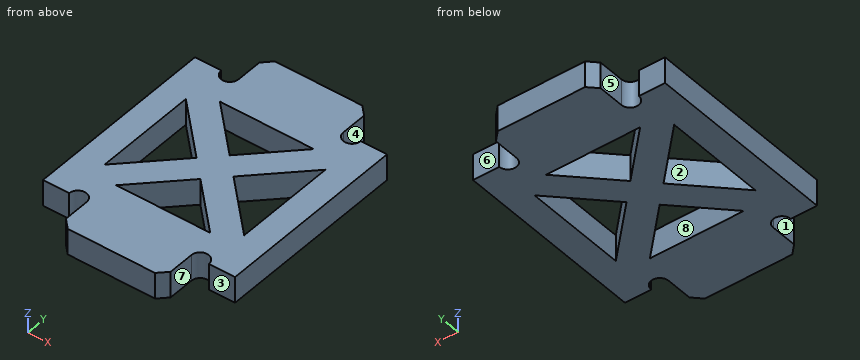
```python
from build123d import *

# Parameters (mm, degrees)
EXTRUDE_1_DEPTH = 1.5
CHAMFER_1_SIZE  = 1


with BuildPart() as part:
    # 草图1 → 凸台-拉伸1 (new, symmetric)
    with BuildSketch(Plane.XY):
        with BuildLine():
            Line((-6, 15), (-6, 11))
            ThreePointArc((-6, 11), (-7, 10), (-8, 11))
            Line((-8, 11), (-11, 11))
            Line((-11, 11), (-11, -11))
            Line((-11, -11), (-8, -11))
            ThreePointArc((-8, -11), (-7, -10), (-6, -11))
            Line((-6, -11), (-6, -15))
            Line((-6, -15), (6, -15))
            Line((6, -15), (6, -11))
            ThreePointArc((6, -11), (7, -10), (8, -11))
            Line((8, -11), (11, -11))
            Line((11, -11), (11, 11))
            Line((11, 11), (8, 11))
            ThreePointArc((8, 11), (7, 10), (6, 11))
            Line((6, 11), (6, 15))
            Line((6, 15), (-6, 15))
        make_face()
        Polygon((5.378679656, 7.5), (0, 2.121320344), (-5.378679656, 7.5), align=None, mode=Mode.SUBTRACT)
        Polygon((0, -2.121320344), (5.378679656, -7.5), (-5.378679656, -7.5), align=None, mode=Mode.SUBTRACT)
        Polygon((-8, 5.878679656), (-2.121320344, 0), (-8, -5.878679656), align=None, mode=Mode.SUBTRACT)
        Polygon((8, -5.878679656), (2.121320344, 0), (8, 5.878679656), align=None, mode=Mode.SUBTRACT)
    extrude(amount=EXTRUDE_1_DEPTH, both=True)

    # 倒角1
    chamfer_1_edges = [part.edges().sort_by_distance(p)[0] for p in [
        (-6, 15, 0),
        (6, 15, 0),
        (6, -15, 0),
        (-6, -15, 0),
    ]]
    chamfer(chamfer_1_edges, length=CHAMFER_1_SIZE)


solid = part.part
```
Work out the finished part from the listing and answer in its coordinate system (mm). Face numbers are marked on the shaded views. A direction names the side the tool comes from. Round coordinates to 2 decimals unless told otherwise and drop trailing zeros. Loops run counter-clockwise (first coordinate to the right, second up) from the corner with the lowest first, then second, coordinate; pieces in that order, holes last. Notation, with made-up numbers: M 51,-35.75 L 75,-35.75 A21 cw 75,-6.75 Z; hole C 37.5,75.5 d3. An arc over 180 degrees is marked long. Use CSV: the item, a comma, the result in double quotes.
Q1. The mould has two halves that part along Y. Classify the marked faces 6, 7 and 8: pulls with the +Y half, pulls with the -Y half, needs draft (parallel to the pull), parting line crosses it, or undercut.
Determined:
face 6,"pulls with the +Y half"
face 7,"needs draft"
face 8,"undercut"
Q2. Section C-C, the plane y = 6.5 is taken. Determine the outline of the cut face in (x, z), then the cut area to 3 significant figures.
Determined:
outline,"M -11,-1.5 L -4.38,-1.5 L -4.38,1.5 L -11,1.5 Z; M 4.38,-1.5 L 11,-1.5 L 11,1.5 L 4.38,1.5 Z"
area,"39.7 mm2"
Q3. Consider L1, parallel to Y at x = 1.75, z = -1.25; L2, parallel to Y at x = 2, z = -0.75; L3, parallel to Y at x = -3.25, z = -0.7. Determine where each line is inside the solid, lowest interval first.
Determined:
L1,"-15 to -7.5, -3.87 to 3.87, 7.5 to 15"
L2,"-15 to -7.5, -4.12 to 4.12, 7.5 to 15"
L3,"-15 to -7.5, -5.37 to -1.13, 1.13 to 5.37, 7.5 to 15"
Q4. A tool of negligible diameter and unlimited length cuts with its end or side. For the marked faces 1, 2, 3, 4 and 5, from which of +Z, -Z, +X, -X, +Y, -Y can it reach the whole face along a straight path? Write none if from no direction.
Determined:
face 1,"+Z, -Z, -X, -Y"
face 2,"+Z, -Z"
face 3,"+Z, -Z, +X, -Y"
face 4,"+Z, -Z, +X, +Y"
face 5,"+Z, -Z, -X, +Y"
Q5. Section A-A, the plane x = -7 is taken. Determine the outline of the cut face in (y, z).
Determined:
outline,"M -10,-1.5 L -4.88,-1.5 L -4.88,1.5 L -10,1.5 Z; M 4.88,-1.5 L 10,-1.5 L 10,1.5 L 4.88,1.5 Z"
Q6. Each of these flat-tipped pins is pushed along its axis until it touches: pin 1 (0.9 mm diameter, centred on y = 12.5, z = 0, fed in from -X); pin 2 (1.5 mm diameter, centred on y = -13, z = 0.5, fed in from +X); pin 3 (1 mm diameter, centred on x = -8.5, z = -1, fed in from +Y). Where does it stop, or does it pass through?
Determined:
pin 1,"x = -6"
pin 2,"x = 6"
pin 3,"y = 11"
Q7. Section B-B, the plane z = 0.7 is taken. State how many separate pieces and enclosed holes the cut face has, then the cut area to 3 significant figures.
Determined:
separate pieces,"1"
enclosed holes,"4"
area,"445 mm2"
Q8. Section D-D, the plane x = 1 is taken. Determine the outline of the cut face in (y, z), then the cut area to 3 significant figures.
Determined:
outline,"M -15,-1.5 L -7.5,-1.5 L -7.5,1.5 L -15,1.5 Z; M -3.12,-1.5 L 3.12,-1.5 L 3.12,1.5 L -3.12,1.5 Z; M 7.5,-1.5 L 15,-1.5 L 15,1.5 L 7.5,1.5 Z"
area,"63.7 mm2"
